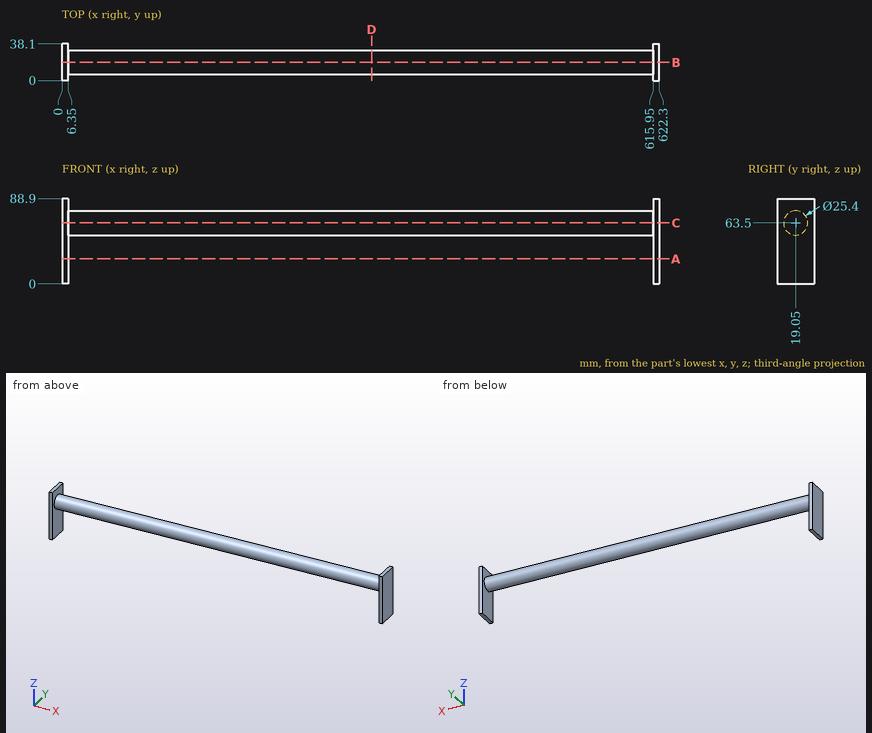
Drawing for the job (mm, zero at the part's lowest x, y, z). Round coordinates to 2 decimals unless told otherwise and drop trailing zeros. Order: outer loops, then holes, each group sorted by start corner. A loop starts at its lowest first (then second) coordinate and runs counter-clockwise, first axis right, second up.
Item 1: Saw through at B-B on y = 19.05. Write the cut outline in (x, z), then the cut area to 3 significant figures.
Item 2: Saw through at C-C on z = 63.5. Write the cut outline in (x, y), then the cut area to 3 significant figures.
Item 3: Saw through at A-A on z = 26. Write the cut outline in (x, y).
Item 4: Pin check, flat tips, straight feed: pin 1 (3 mm diameter, centred on x = 137, y = 21, fed in from -Z); pin 2 (8 mm diameter, centred on x = 177, z = 70.5, fed in from +Y); pin 3 (5 mm diameter, centred on x = 466.5, y = 10, fed in from +Z). Stop position of each tip, or through.
Item 5: Saw through at D-D on x = 322.5. Write the cut outline in (y, z).
Item 6: Probe line 1 along X through (y, z) = (26, 46.5); line 2 along Y through (x, z) = (59, 59.5); line 3 along Y through (x, z) = (239, 64). List the from-to ranges inside material, lowest first.
Reported:
1. outline: (0, 0) - (6.35, 0) - (6.35, 50.8) - (615.95, 50.8) - (615.95, 0) - (622.3, 0) - (622.3, 88.9) - (615.95, 88.9) - (615.95, 76.2) - (6.35, 76.2) - (6.35, 88.9) - (0, 88.9) - close
1. area: 16,600 mm2
2. outline: (0, 0) - (6.35, 0) - (6.35, 6.35) - (615.95, 6.35) - (615.95, 0) - (622.3, 0) - (622.3, 38.1) - (615.95, 38.1) - (615.95, 31.75) - (6.35, 31.75) - (6.35, 38.1) - (0, 38.1) - close
2. area: 16,000 mm2
3. outline: (0, 0) - (6.35, 0) - (6.35, 38.1) - (0, 38.1) - close; (615.95, 0) - (622.3, 0) - (622.3, 38.1) - (615.95, 38.1) - close
4. pin 1: stops at z = 50.81
4. pin 2: stops at y = 31.39
4. pin 3: stops at z = 74.38
5. outline: circle Ø25.4 at (19.05, 63.5)
6. line 1: x = 0 to 6.35, 615.95 to 622.3
6. line 2: y = 7 to 31.1
6. line 3: y = 6.36 to 31.74
